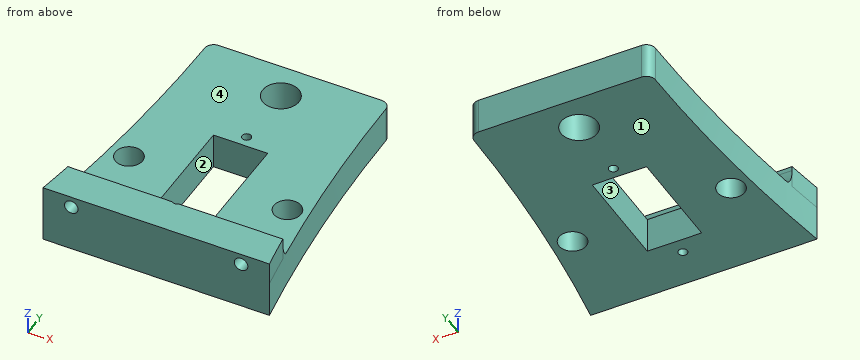
```python
from build123d import *

# Parameters (mm, degrees)
BOSS_EXTRUDE1_DEPTH  = 8
BOSS_EXTRUDE2_DEPTH  = 5
SKETCH3_R            = 1.5
CUT_EXTRUDE_DEPTH    = 8
FILLET1_SIZE         = 4
FILLET1_SIZE_2       = 2
FILLET2_R            = 2
SKETCH4_R            = 4.0005
SKETCH4_R_2          = 4.725
SKETCH4_R_3          = 3
M4_H6_T_INSERT_DEPTH = 8
SKETCH12_R           = 1
SKETCH12_W           = 12
SKETCH12_H           = 23
CUT_EXTRUDE1_DEPTH   = 67.287253734


with BuildPart() as part:
    # Sketch1 → Boss-Extrude1 (new body)
    with BuildSketch(Plane.XY):
        with BuildLine():
            Line((20, 60), (-20, 60))
            ThreePointArc((-20, 60), (-21.252162636, 29.896013553), (-25, 0))
            Line((-25, 0), (25, 0))
            ThreePointArc((25, 0), (21.252162636, 29.896013553), (20, 60))
        make_face()
    extrude(amount=BOSS_EXTRUDE1_DEPTH)

    # Sketch2 → Boss-Extrude2 (add)
    with BuildSketch(Plane.XY.offset(8)):
        with BuildLine():
            Line((-25, 0), (25, 0))
            ThreePointArc((25, 0), (24.352183064, 3.996507037), (23.749041813, 8))
            Line((23.749041813, 8), (-23.749041813, 8))
            ThreePointArc((-23.749041813, 8), (-24.352183064, 3.996507037), (-25, 0))
        make_face()
    extrude(amount=BOSS_EXTRUDE2_DEPTH)

    # Sketch3 → Cut-Extrude (cut)
    with BuildSketch(Plane(origin=(0, 8, 0), x_dir=(1, 0, 0), z_dir=(0, 1, 0))):
        with Locations(Location((-18.749041813, -10.5, 0), (0, 0, 270))):
            Circle(SKETCH3_R)
        with Locations(Location((18.749041813, -10.5, 0), (0, 0, 270))):
            Circle(SKETCH3_R)
    extrude(amount=-CUT_EXTRUDE_DEPTH, mode=Mode.SUBTRACT)

    # Fillet1
    # an asymmetric fillet: 4, 2 mm, written as the material it adds along each edge
    with BuildSketch(Plane(origin=(33.749041813, 8, 8), x_dir=(0, 0, 1), z_dir=(-1, 0, 0))) as fillet1_piece_1_section:
        with BuildLine():
            Bezier((FILLET1_SIZE, 0), (0, 0), (0, FILLET1_SIZE_2), weights=[1, 0.707106781, 1])
            Line((0, FILLET1_SIZE_2), (-0.08, 2))
            Line((-0.08, 2), (-0.08, -0.08))
            Line((-0.08, -0.08), (4, -0.08))
            Line((4, -0.08), (FILLET1_SIZE, 0))
        make_face()
    fillet1_piece_1 = extrude(amount=67.498083626, mode=Mode.PRIVATE)
    fillet1_piece_1 = fillet1_piece_1 - Plane(origin=(382.5, 60, 8.944071766), x_dir=(-0.9862068965517241, -0.1655172413793104, 0), z_dir=(0, 0, -1)) * Cylinder(362.5, 151, mode=Mode.PRIVATE)
    fillet1_piece_1 = fillet1_piece_1 - Plane(origin=(-382.5, 60, 8.944071766), x_dir=(1, 0, 0), z_dir=(0, 0, -1)) * Cylinder(362.5, 151, mode=Mode.PRIVATE)
    fillet1_piece_1 = fillet1_piece_1 - Plane(origin=(-18.749041813, 8.425382089, 10.5), x_dir=(0, 0, 1), z_dir=(0, 1, 0)) * Cylinder(1.5, 151, mode=Mode.PRIVATE)
    fillet1_piece_1 = fillet1_piece_1 - Plane(origin=(18.749041813, 8.425382089, 10.5), x_dir=(0, 0, 1), z_dir=(0, 1, 0)) * Cylinder(1.5, 151, mode=Mode.PRIVATE)
    add(fillet1_piece_1)

    # Fillet2
    fillet2_edges = [part.edges().sort_by_distance(p)[0] for p in [
        (20, 60, 4),
        (-20, 60, 4),
    ]]
    fillet(fillet2_edges, radius=FILLET2_R)

    # Sketch4 → M4*H6 T-Insert (cut)
    with BuildSketch(Plane(origin=(0, 0, 0), x_dir=(-1, 0, 0), z_dir=(0, 0, -1))):
        with Locations((0, 52)):
            Circle(SKETCH4_R)
        with Locations((0, 29.37)):
            Circle(SKETCH4_R_2)
        with Locations((-17.5, 21.695)):
            Circle(SKETCH4_R_3)
        with Locations(Location((17.5, 21.695, 0), (0, 0, 180))):
            Circle(SKETCH4_R_3)
    extrude(amount=-M4_H6_T_INSERT_DEPTH, mode=Mode.SUBTRACT)

    # Sketch12 → Cut-Extrude1 (cut, through all)
    with BuildSketch(Plane(origin=(0, 0, 0), x_dir=(-1, 0, 0), z_dir=(0, 0, -1))):
        with Locations((0, 37.72)):
            Circle(SKETCH12_R)
        with Locations(Location((0, 8.72, 0), (0, 0, 313.945519562))):
            Circle(SKETCH12_R)
        with Locations((0, 23.72)):
            Rectangle(SKETCH12_W, SKETCH12_H)
    extrude(amount=-CUT_EXTRUDE1_DEPTH, mode=Mode.SUBTRACT)


solid = part.part
```
CAD build for the part. Positions are in the model's coordinates, mm. Face numbers are marked on the shaded views. A direction names the side the tool comes from. Give positions to 0.01 mm unless a question says otherwise; leave off trailing zeros. Loops run counter-clockwise (first coordinate to the right, second up) from the corner with the lowest first, then second, coordinate; pieces in that order, holes last. Notation, with made-up numbers: (-30, 37.5) -> (2, 37.5) arc R30 ccw to (2, 73.5) -> close; hole circle Ø2 at (10, 6). An arc over 180 degrees is marked (long way). Use a Markdown table: item, result.
1. Slice it at A-A (y = 37.72). List the corners of the cut face in (x, z).
Check result:
| item | result |
|---|---|
| outline | (-20.69, 0) -> (-1, 0) -> (-1, 8) -> (-20.69, 8) -> close; (1, 0) -> (20.69, 0) -> (20.69, 8) -> (1, 8) -> close |
2. Wall check: L1, parallel to Y at x = -17.5, z = 5.25 (3 decimals); L2, parallel to Y at x = 0, z = 5; L3, parallel to X at y = 5.5, z = 10.5. Give the ranges that are in metal, low to high. Write a range as [from, to].
Check result:
| item | result |
|---|---|
| L1 | y = [0, 18.695], [24.695, 60] |
| L2 | y = [0, 7.72], [9.72, 12.22], [35.22, 36.72], [38.72, 48], [56, 60] |
| L3 | x = [-24.12, -20.25], [-17.25, 17.25], [20.25, 24.12] |
3. Slice it at D-D (y = 6). List the corners of the cut face in (x, z), plus the area to 3 significant figures.
Check result:
| item | result |
|---|---|
| outline | (-24.04, 0) -> (24.04, 0) -> (24.04, 13) -> (-24.04, 13) -> close; hole circle Ø3 at (-18.75, 10.5); hole circle Ø3 at (18.75, 10.5) |
| area | 611 mm^2 |
4. Which spindle directions (+Z, -Z, +X, -X, +Y, -Y) get a long thin tool onto all of the face, cutting with end or side? Do the marked faces 1 and 2. Say none if no direction does.
Check result:
| item | result |
|---|---|
| face 1 | -Z, +X, -X, +Y, -Y |
| face 2 | +Z, -Z |
5. Slice it at B-B (y = 21). List the corners of the cut face in (x, z), plus the area to 3 significant figures.
Check result:
| item | result |
|---|---|
| outline | (-22.1, 0) -> (-20.42, 0) -> (-20.42, 8) -> (-22.1, 8) -> close; (-14.58, 0) -> (-6, 0) -> (-6, 8) -> (-14.58, 8) -> close; (6, 0) -> (14.58, 0) -> (14.58, 8) -> (6, 8) -> close; (20.42, 0) -> (22.1, 0) -> (22.1, 8) -> (20.42, 8) -> close |
| area | 164 mm^2 |
6. Flat gauge pins, fed straight in: pin 1 (2 mm diameter, centred on x = 8.5, y = 28, fed in from +Z); pin 2 (1.6 mm diameter, centred on x = 0, y = 37.72, fed in from -Z); pin 3 (4 mm diameter, centred on y = 26, z = 3.5, fed in from -X); pin 4 (0.5 mm diameter, centred on x = 7, z = 12.5, fed in from +Y). Where does each tip first touch, or does it go through?
Check result:
| item | result |
|---|---|
| pin 1 | stops at z = 8 |
| pin 2 | passes through |
| pin 3 | stops at x = -21.79 |
| pin 4 | stops at y = 8 |
7. Slice it at C-C (z = 7.25). List the corners of the cut face in (x, y) (1 decimal), plus the area to 3 significant figures.
Check result:
| item | result |
|---|---|
| outline | (-25, 0) -> (25, 0) arc R362.5 cw to (20, 58) arc R2 ccw to (18, 60) -> (-18, 60) arc R2 ccw to (-20, 58) arc R362.5 cw to start; hole circle Ø6 at (-17.5, 21.7); hole (-6, 12.2) -> (6, 12.2) -> (6, 35.2) -> (-6, 35.2) -> close; hole circle Ø8 at (0, 52); hole circle Ø2 at (0, 8.7); hole circle Ø2 at (0, 37.7); hole circle Ø6 at (17.5, 21.7) |
| area | 2,210 mm^2 |
8. Mould opens along X. For the marked faces 3 and 4 say: pulls with the +X half, pulls with the -X half, needs draft (parallel to the pull), parting line crosses it, or undercut.
Check result:
| item | result |
|---|---|
| face 3 | undercut |
| face 4 | needs draft |
